```python
from build123d import *

# Parameters (mm, degrees)
SKETCH1_W           = 50.8
SKETCH1_H           = 50.8
BOSS_EXTRUDE2_DEPTH = 3.175


with BuildPart() as part:
    # Sketch1 → Boss-Extrude2 (new body)
    with BuildSketch(Plane.XY):
        with Locations((25.4, -25.4)):
            Rectangle(SKETCH1_W, SKETCH1_H)
    extrude(amount=BOSS_EXTRUDE2_DEPTH)

    # Sketch2 → 1/4 (0.25) Diameter Hole1 (revolve, cut)
    with BuildSketch(Plane(origin=(28.083631343, -27.305207035, 0), x_dir=(0, 1, 0), z_dir=(1, 0, 0))):
        Polygon((0, 0), (0, 3.175), (3.175, 3.175), (3.175, 4.090710056), (6.731, 0), align=None)
    revolve(axis=Axis((28.083631343, -27.305207035, -6.35), (0, 0, 1)), mode=Mode.SUBTRACT)


solid = part.part
```
Check sheet for the modelled part. Datum: model origin and axes. Units: mm. Give positions to 0.01 mm unless a question says otherwise; leave off trailing zeros. Write each loop counter-clockwise with the first axis right and the second up, starting at its lowest first coordinate (ties: lowest second). Pieces come first, ordered by that corner, then holes. Notation, with made-up numbers: (-37, 64) -> (21, 64) arc R28 cw to (21, 90) -> close; hole circle Ø11 at (89, -17). An arc over 180 degrees is marked (long way). Use CSV: the item, a comma, the result in double quotes. Start each with the question number.
Q1. Scan lines: line 1 along Y through (x, z) = (32, 1.85); line 2 along Y through (x, z) = (27, 1.4); line 3 along X through (y, z) = (-32, 1.3). Record each from-to range of solid material in increasing order.
Q2. Cross-section at A-A on z = 0.55. Enter the section's corners in (x, y), and give its area (3 significant figures).
Q3. Release check for a two-part mould opening along X. For faces 1 (the conical face through (32.129, -28.203, 2.976)), 2 (the flat face through (19, -25, 3.175)), 3 (the flat face through (50.8, -26, 2)) record: +X half, -X half, draft (parallel to the pull), parting line (faces both ways), or undercut.
Q4. Depth check by flat-ended pin: P1, Ø6, axis at x = 31, y = -27, coming from the -Z side. Enter the tip coordinate at first touch or a pass-through.
Working result:
1,line 1,"y = -50.8 to -30.61, -24 to 0"
1,line 2,"y = -50.8 to -32.71, -21.9 to 0"
1,line 3,"x = 0 to 25.03, 31.14 to 50.8"
2,outline,"(0, -50.8) -> (50.8, -50.8) -> (50.8, 0) -> (0, 0) -> close; hole circle Ø12.51 at (28.08, -27.31)"
2,area,"2,460 mm^2"
3,face 1,"undercut"
3,face 2,"draft"
3,face 3,"+X half"
4,P1,"stops at z = 0.92"
